Build history of the part. All positions in model axes, mm. Give positions to 0.01 mm unless a question says otherwise; leave off trailing zeros. Loops run counter-clockwise (first coordinate to the right, second up) from the corner with the lowest first, then second, coordinate; pieces in that order, holes last. Notation, with made-up numbers: M -3.75,62 L 49.25,62 A20 cw 49.25,67 Z; hole C 4,54.5 d10. An arc over 180 degrees is marked long. Answer as a JSON object with one key per item and string values. Group by question number.
1. Slice it at C-C (x = 40). List the corners of the cut face in (y, z), then the cut area to 3 significant figures.
2. Slice it at D-D (y = 0.7). List the corners of the cut face in (x, z).
3. Slice it at B-B (z = 0). List the corners of the cut face in (x, y), then the cut area to 3 significant figures.
4. Drop flat-ended pins along their axis: pin 1 Ø0.8 at (x, y) = (1.5, 1) entering from +Z; pin 2 Ø4 at (x, z) = (-67.5, 56.5) entering from -Y; pin 3 Ø0.8 at (y, z) = (1.5, 17.5) entering from +X; pin 4 Ø0.8 at (x, y) = (14, 1) entering from -Z. Give the stop position or say it passes through.
5. Drill centre lines: line 1 along X through (y, z) = (1.95, 0); line 2 along Z through (x, y) = (44.5, 2.05); line 3 along Z through (x, y) = (37.5, 1.7). Where is each one in solid material? Low to high. Write a range as [from, to].
6. Slice it at A-A (x = 0). List the corners of the cut face in (y, z).
from build123d import *

# Parameters (mm, degrees)
SKETCH1_R           = 88.519
SKETCH1_W           = 104.14
SKETCH1_H           = 104.14
BOSS_EXTRUDE1_DEPTH = 2.54
SKETCH2_R           = 6.35
CUT_EXTRUDE1_DEPTH  = 126.210535986


with BuildPart() as part:
    # Sketch1 → Boss-Extrude1 (new body)
    with BuildSketch(Plane(origin=(0, 0, 0), x_dir=(1, 0, 0), z_dir=(0, 1, 0))):
        with Locations(Location((0, 0, 0), (0, 0, 270))):
            Circle(SKETCH1_R)
        Rectangle(SKETCH1_W, SKETCH1_H, mode=Mode.SUBTRACT)
    extrude(amount=BOSS_EXTRUDE1_DEPTH)

    # Sketch2 → Cut-Extrude1 (cut, through all)
    with BuildSketch(Plane(origin=(0, 2.54, 0), x_dir=(1, 0, 0), z_dir=(0, 1, 0))):
        with Locations(Location((0, 70.358, 0), (0, 0, 270))):
            Circle(SKETCH2_R)
        with Locations(Location((70.358, 0, 0), (0, 0, 270))):
            Circle(SKETCH2_R)
        with Locations(Location((0, -70.358, 0), (0, 0, 270))):
            Circle(SKETCH2_R)
        with Locations(Location((-70.358, 0, 0), (0, 0, 270))):
            Circle(SKETCH2_R)
    extrude(amount=-CUT_EXTRUDE1_DEPTH, mode=Mode.SUBTRACT)


solid = part.part
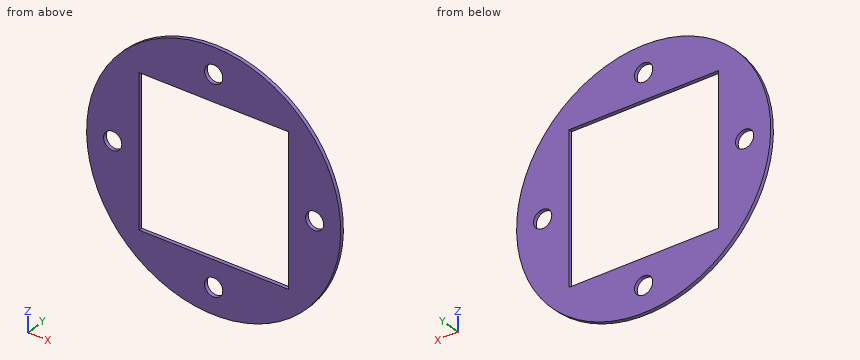
Established:
{
 "1": {"outline": "M 0,-78.97 L 2.54,-78.97 L 2.54,-52.07 L 0,-52.07 Z; M 0,52.07 L 2.54,52.07 L 2.54,78.97 L 0,78.97 Z", "area": "137 mm^2"},
 "2": {"outline": "C 0,0 d177.04; hole C -70.36,0 d12.7; hole M -52.07,-52.07 L 52.07,-52.07 L 52.07,52.07 L -52.07,52.07 Z; hole C 0,-70.36 d12.7; hole C 0,70.36 d12.7; hole C 70.36,0 d12.7"},
 "3": {"outline": "M -88.52,0 L -76.71,0 L -76.71,2.54 L -88.52,2.54 Z; M -64.01,0 L -52.07,0 L -52.07,2.54 L -64.01,2.54 Z; M 52.07,0 L 64.01,0 L 64.01,2.54 L 52.07,2.54 Z; M 76.71,0 L 88.52,0 L 88.52,2.54 L 76.71,2.54 Z", "area": "121 mm^2"},
 "4": {"pin 1": "stops at z = 88.51", "pin 2": "stops at y = 0", "pin 3": "stops at x = 86.85", "pin 4": "stops at z = -87.47"},
 "5": {"line 1": "x = [-88.52, -76.71], [-64.01, -52.07], [52.07, 64.01], [76.71, 88.52]", "line 2": "z = [-76.52, -52.07], [52.07, 76.52]", "line 3": "z = [-80.18, -52.07], [52.07, 80.18]"},
 "6": {"outline": "M 0,-88.52 L 2.54,-88.52 L 2.54,-76.71 L 0,-76.71 Z; M 0,-64.01 L 2.54,-64.01 L 2.54,-52.07 L 0,-52.07 Z; M 0,52.07 L 2.54,52.07 L 2.54,64.01 L 0,64.01 Z; M 0,76.71 L 2.54,76.71 L 2.54,88.52 L 0,88.52 Z"}
}
